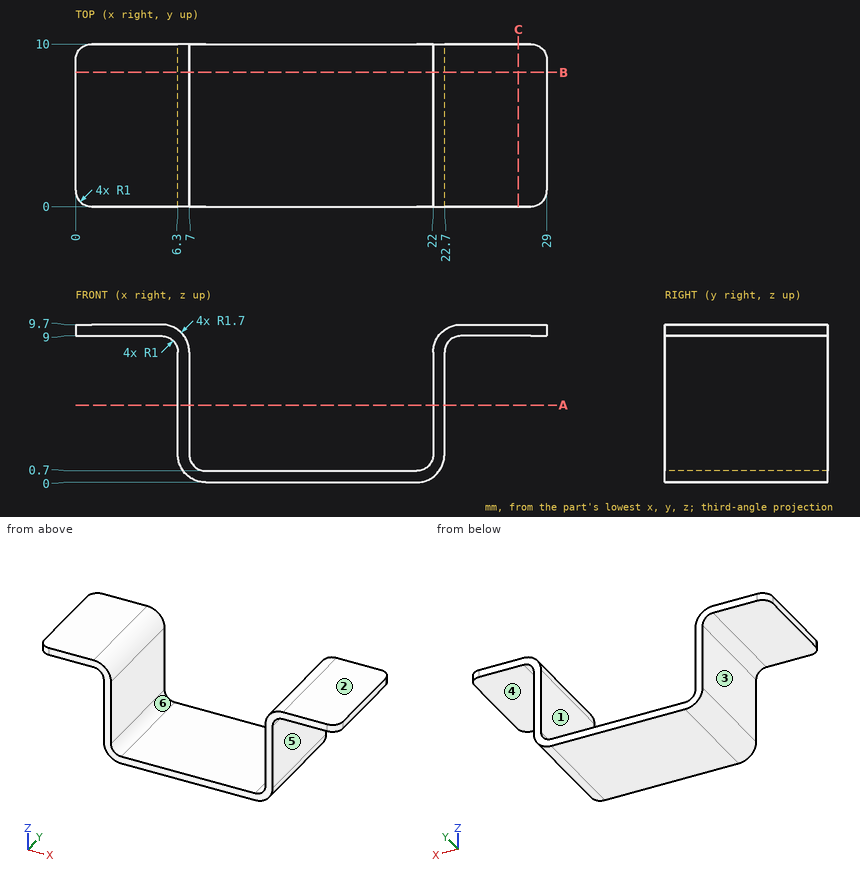
Geometry check sheet. Reference: drawing and pictorial views, mm from the part's lowest x, y, z. A direction names the side the tool comes from. Give positions to 0.01 mm unless a question says otherwise; leave off trailing zeros. Loops run counter-clockwise (first coordinate to the right, second up) from the corner with the lowest first, then second, coordinate; pieces in that order, holes last. Notation, with made-up numbers: (1.5, 14.5) - (55.5, 14.5) arc R28 ccw to (55.5, 39.5) - close; hole circle Ø4 at (-25.5, -6.5). An arc over 180 degrees is marked (long way). One line per question, with ' | ' between items. Start each with the question number.
1. Draft check along X on the marked faces 4, 5 and 6. Enter one of: released by +X, released by -X, zero draft, split by the parting line, or undercut.
2. Set-up check for the marked faces 1, 2 and 3: record each of +Z, -Z, +X, -X, +Y, -Y from which the full face is reachable in a straight line by a thin tool's end or side.
3. Cross-section at C-C, the plane x = 27.25. Enter the section's corners in (y, z), plus the area to 3 significant figures.
4. Cross-section at B-B, the plane y = 8.25. Enter the section's corners in (x, z).
5. Gauge pin test, flat ends, axial feed: pin 1 Ø3 at (y, z) = (3, 5) entering from +X; pin 2 Ø1.5 at (x, y) = (15, 8.5) entering from +Z; pin 3 Ø2.5 at (x, y) = (26, 2.5) entering from -Z. Record the tip position at first contact, or that the pin passes through.
6. Material ranges on line 1 along X through (y, z) = (3.75, 3.5); line 2 along Z through (x, y) = (25.75, 9.5); line 3 along Z through (x, y) = (10.5, 1), recorded low to high. Write a range as [from, to].
7. Cross-section at A-A, the plane z = 4.75. Enter the section's corners in (x, y).
Check result:
1) face 4: zero draft | face 5: released by +X | face 6: undercut
2) face 1: +Z, +Y, -Y | face 2: +Z, +X, -X, +Y, -Y | face 3: -Z, -X, +Y, -Y
3) outline: (0, 9) - (10, 9) - (10, 9.7) - (0, 9.7) - close | area: 7.00 mm2
4) outline: (0, 9) - (5.3, 9) arc R1 cw to (6.3, 8) - (6.3, 1.7) arc R1.7 ccw to (8, 0) - (21, 0) arc R1.7 ccw to (22.7, 1.7) - (22.7, 8) arc R1 cw to (23.7, 9) - (29, 9) - (29, 9.7) - (23.7, 9.7) arc R1.7 ccw to (22, 8) - (22, 1.7) arc R1 cw to (21, 0.7) - (8, 0.7) arc R1 cw to (7, 1.7) - (7, 8) arc R1.7 ccw to (5.3, 9.7) - (0, 9.7) - close
5) pin 1: stops at x = 22.7 | pin 2: stops at z = 0.7 | pin 3: stops at z = 9
6) line 1: x = [6.3, 7], [22, 22.7] | line 2: z = [9, 9.7] | line 3: z = [0, 0.7]
7) outline: (6.3, 0) - (7, 0) - (7, 10) - (6.3, 10) - close; (22, 0) - (22.7, 0) - (22.7, 10) - (22, 10) - close
